Read the model definition and answer for the solid it produces. Units are mm, in the model's axes. Face numbers are marked on the shaded views. A direction names the side the tool comes from. Give positions to 0.01 mm unless a question says otherwise; leave off trailing zeros. Write each loop counter-clockwise with the first axis right and the second up, starting at its lowest first coordinate (ties: lowest second). Pieces come first, ordered by that corner, then holes. Notation, with made-up numbers: (15, 60.25) -> (37, 60.25) arc R22 cw to (37, 68.25) -> close; hole circle Ø5 at (21, 8). An arc over 180 degrees is marked (long way). Use a Markdown table: item, result.
from build123d import *

# Parameters (mm, degrees)
F0_R     = 12.573
F1_DEPTH = 15.4686
F2_R     = 9.398
F3_DEPTH = 3.048
F4_SIZE  = 0.762
F5_R     = 3
F6_DEPTH = 6.35


with BuildPart() as f1:
    # F0 (on Front) → F1 (new body)
    with BuildSketch(Plane.XZ):
        Circle(F0_R)
    extrude(amount=F1_DEPTH)

    # F2 (on face) → F3 (cut)
    with BuildSketch(Plane(origin=(0, 0, 0), x_dir=(-1, 0, 0), z_dir=(0, 1, 0))):
        Circle(F2_R)
    extrude(amount=-F3_DEPTH, mode=Mode.SUBTRACT)

    # F4
    f4_edges = [f1.edges().sort_by_distance(p)[0] for p in [
        (-12.573, -15.4686, 0),
    ]]
    chamfer(f4_edges, length=F4_SIZE)

    # F5 (on face) → F6 (join)
    with BuildSketch(Plane(origin=(0, -3.048, 0), x_dir=(-1, 0, 0), z_dir=(0, 1, 0))):
        Circle(F5_R)
    extrude(amount=F6_DEPTH)


solid = f1.part
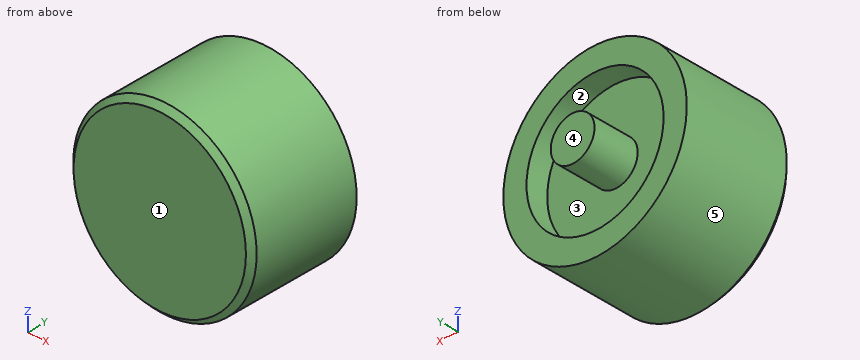
Item 1: A cutting plane is placed at B-B (z = 0). Give the vertices of the cut face in (x, y).
Return value:
| item | result |
|---|---|
| outline | (-12.57, -14.71) -> (-11.81, -15.47) -> (11.81, -15.47) -> (12.57, -14.71) -> (12.57, 0) -> (9.4, 0) -> (9.4, -3.05) -> (3, -3.05) -> (3, 3.3) -> (-3, 3.3) -> (-3, -3.05) -> (-9.4, -3.05) -> (-9.4, 0) -> (-12.57, 0) -> close |
Item 2: A cutting plane is placed at D-D (y = -4). Give the vertices of the cut face in (x, z).
Return value:
| item | result |
|---|---|
| outline | circle Ø25.15 at (0, 0) |
Item 3: A cutting plane is placed at A-A (y = -1.5). Give the vertices of the cut face in (x, z), then the cut area to 3 significant figures.
Return value:
| item | result |
|---|---|
| outline | circle Ø25.15 at (0, 0); circle Ø6 at (0, 0); hole circle Ø18.8 at (0, 0) |
| area | 247 mm^2 |
Item 4: Each of these flat-tipped pins is pushed along its axis until it touches: P1, Ø3, axis at x = -5.5, y = -12, coming from the -Z side; P2, Ø3, axis at x = 10, y = -10.5, coming from the -Z side; P3, Ø1.5, axis at x = 7, z = -3, coming from the +Y side. Where does it stop, or does it pass through?
Return value:
| item | result |
|---|---|
| P1 | z = -11.92 |
| P2 | z = -9.26 |
| P3 | y = -3.05 |
Item 5: A tool of negligible diameter and unlimited length cuts with its end or side. For the marked faces 1 and 2, from which of +Z, -Z, +X, -X, +Y, -Y can it reach the whole face along a straight path? Write none if from no direction.
Return value:
| item | result |
|---|---|
| face 1 | +Z, -Z, +X, -X, -Y |
| face 2 | +Y |
Item 6: For a pull along X with two mould halves and no side action, classify the marked faces 3, 4 and 5 as +X half, -X half, draft (parallel to the pull), parting line (faces both ways), or undercut.
Return value:
| item | result |
|---|---|
| face 3 | undercut |
| face 4 | draft |
| face 5 | parting line |
Item 7: A cutting plane is placed at C-C (x = 0). Give the vertices of the cut face in (y, z), then the cut area to 3 significant figures.
Return value:
| item | result |
|---|---|
| outline | (-15.47, -11.81) -> (-14.71, -12.57) -> (0, -12.57) -> (0, -9.4) -> (-3.05, -9.4) -> (-3.05, -3) -> (3.3, -3) -> (3.3, 3) -> (-3.05, 3) -> (-3.05, 9.4) -> (0, 9.4) -> (0, 12.57) -> (-14.71, 12.57) -> (-15.47, 11.81) -> close |
| area | 369 mm^2 |
Item 8: Straight lines are drawn through the part: line 1 along Z through (x, y) = (0, -1.15); line 2 along Z through (x, y) = (1.25, -2.75); line 3 along Y through (x, z) = (-0.75, -7.5). For each, find the intervals that lie inside material, in ascending order. Write a range as [from, to].
Return value:
| item | result |
|---|---|
| line 1 | [-12.57, -9.4], [-3, 3], [9.4, 12.57] |
| line 2 | [-12.51, -9.31], [-2.73, 2.73], [9.31, 12.51] |
| line 3 | [-15.47, -3.05] |
